Print and shaded views of the part. All mm, measured from the part's lowest x, y and z. Round coordinates to 2 decimals unless told otherwise and drop trailing zeros. Write each loop counter-clockwise with the first axis right and the second up, starting at its lowest first coordinate (ties: lowest second). Pieces come first, ordered by that corner, then holes. Notation, with made-up numbers: M -26,68 L -16,68 A29 ccw -16,103 Z; hole C 80,19 d9. An arc over 180 degrees is marked long. Write item = value, one per line. Start each with the question number.
Q1. Band-saw the part on C-C on z = 0.65. Write the cut outline in (x, y) (3 decimals).
Q2. Band-saw the part on A-A on x = 4.5. Write the cut outline in (y, z) (3 decimals), plus the area to 3 significant figures.
Q3. Drop a flat-ended pin along its axis: P1, Ø4, axis at x = 14.5, y = 20, coming from the -Z side. Give the stop position or say it passes through.
Q4. Pull direction Y, two halves, no side cores. Call the marked faces 1, 2, 3 and 4: released by +Y, released by -Y, zero draft, split by the parting line, or undercut.
Q5. Band-saw the part on B-B on y = 20. Write the cut outline in (x, z), plus the area to 3 significant figures.
Q6. Probe L1, parallel to Y at x = 4.5, z = 0.85 (3 decimals); L2, parallel to Y at x = 4, z = 1.2; L3, parallel to X at y = 34, z = 0.8. List the from-to ranges inside material, lowest first.
Q7. Band-saw the part on D-D on y = 33. Write the cut outline in (x, z), plus the area to 3 significant figures.
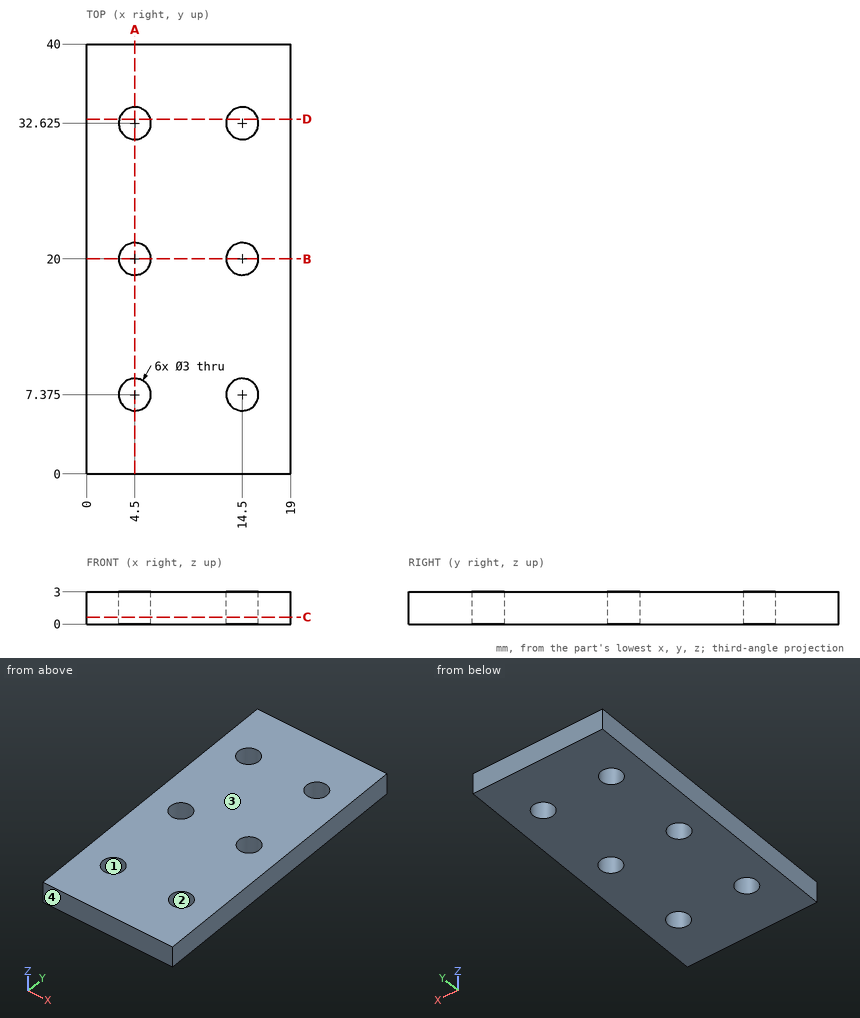
Conclusion:
q1.outline = M 0,0 L 19,0 L 19,40 L 0,40 Z; hole C 4.5,7.375 d3; hole C 4.5,20 d3; hole C 4.5,32.625 d3; hole C 14.5,7.375 d3; hole C 14.5,20 d3; hole C 14.5,32.625 d3
q2.outline = M 0,0 L 5.875,0 L 5.875,3 L 0,3 Z; M 8.875,0 L 18.5,0 L 18.5,3 L 8.875,3 Z; M 21.5,0 L 31.125,0 L 31.125,3 L 21.5,3 Z; M 34.125,0 L 40,0 L 40,3 L 34.125,3 Z
q2.area = 93.0 mm^2
q3.P1 = 0
q4.face_1 = undercut
q4.face_2 = undercut
q4.face_3 = zero draft
q4.face_4 = released by -Y
q5.outline = M 0,0 L 3,0 L 3,3 L 0,3 Z; M 6,0 L 13,0 L 13,3 L 6,3 Z; M 16,0 L 19,0 L 19,3 L 16,3 Z
q5.area = 39.0 mm^2
q6.L1 = 0 to 5.875, 8.875 to 18.5, 21.5 to 31.125, 34.125 to 40
q6.L2 = 0 to 5.96, 8.79 to 18.59, 21.41 to 31.21, 34.04 to 40
q6.L3 = 0 to 3.9, 5.1 to 13.9, 15.1 to 19
q7.outline = M 0,0 L 3.05,0 L 3.05,3 L 0,3 Z; M 5.95,0 L 13.05,0 L 13.05,3 L 5.95,3 Z; M 15.95,0 L 19,0 L 19,3 L 15.95,3 Z
q7.area = 39.6 mm^2
